```python
from build123d import *

# Parameters (mm, degrees)
F1_DEPTH = 12.7
F2_R     = 2.54
F3_DEPTH = 7.62
F4_R     = 3.175
F5_DEPTH = 2.54


# Not quite as in the source:
# - ends of sketch curves that miss each other by under 0.0002 mm in the source are joined


with BuildPart() as f1:
    # F0 (on Front) → F1 (new body)
    with BuildSketch(Plane.XZ):
        with BuildLine():
            Line((-46.1111856, 159.2312536), (-64.7111856, 159.2312536))
            ThreePointArc((-64.7111856, 159.2312536), (-64.9940283125, 159.1140963125), (-65.1111856, 158.8312536))
            Line((-65.1111856, 158.8312536), (-65.1111856, 157.2332636))
            Line((-65.1111856, 157.2332636), (-64.9611856, 157.2332636))
            Line((-64.9611856, 157.2332636), (-64.9611856, 137.6312536))
            Line((-64.9611856, 137.6312536), (-65.1111856, 137.6312536))
            Line((-65.1111856, 137.6312536), (-65.1111856, 135.7900576))
            ThreePointArc((-65.1111856, 135.7900576), (-65.080737413, 135.6369842271), (-64.9940283125, 135.5072148875))
            Line((-64.9940283125, 135.5072148875), (-63.7917726, 134.3049586))
            Line((-63.7917726, 134.3049586), (-64.1453256, 133.9514056))
            Line((-64.1453256, 133.9514056), (-63.6715641479, 133.4776440521))
            Line((-63.6715641479, 133.4776440521), (-59.6693400521, 129.4754191479))
            Line((-59.6693400521, 129.4754191479), (-59.1955786, 129.0016576))
            Line((-59.1955786, 129.0016576), (-58.8420246, 129.3552116))
            Line((-58.8420246, 129.3552116), (-57.6352246, 128.1484116))
            ThreePointArc((-57.6352246, 128.1484116), (-57.5054559729, 128.061701787), (-57.3523826, 128.0312536))
            Line((-57.3523826, 128.0312536), (-46.1111856, 128.0312536))
            ThreePointArc((-46.1111856, 128.0312536), (-44.6969720376, 128.6170400376), (-44.1111856, 130.0312536))
            Line((-44.1111856, 130.0312536), (-44.1111856, 134.1120546))
            Line((-44.1111856, 134.1120546), (-44.1111856, 153.1264526))
            Line((-44.1111856, 153.1264526), (-44.1111856, 156.3312536))
            Line((-44.1111856, 156.3312536), (-44.1111856, 157.2312536))
            ThreePointArc((-44.1111856, 157.2312536), (-44.6969720376, 158.6454671624), (-46.1111856, 159.2312536))
        make_face()
        with BuildLine():
            Line((-49.0111856, 132.4312536), (-47.1111856, 132.4312536))
            ThreePointArc((-47.1111856, 132.4312536), (-46.0505254282, 131.9919137718), (-45.6111856, 130.9312536))
            ThreePointArc((-45.6111856, 130.9312536), (-46.0505254282, 129.8705934282), (-47.1111856, 129.4312536))
            Line((-47.1111856, 129.4312536), (-49.0111856, 129.4312536))
            ThreePointArc((-49.0111856, 129.4312536), (-50.0718457718, 129.8705934282), (-50.5111856, 130.9312536))
            ThreePointArc((-50.5111856, 130.9312536), (-50.0718457718, 131.9919137718), (-49.0111856, 132.4312536))
        make_face(mode=Mode.SUBTRACT)
        with BuildLine():
            ThreePointArc((-47.1111856, 157.8312536), (-46.0505254282, 157.3919137718), (-45.6111856, 156.3312536))
            ThreePointArc((-45.6111856, 156.3312536), (-46.0505254282, 155.2705934282), (-47.1111856, 154.8312536))
            ThreePointArc((-47.1111856, 154.8312536), (-48.1718457718, 155.2705934282), (-48.6111856, 156.3312536))
            ThreePointArc((-48.6111856, 156.3312536), (-48.1718457718, 157.3919137718), (-47.1111856, 157.8312536))
        make_face(mode=Mode.SUBTRACT)
    extrude(amount=F1_DEPTH)

    # F2 (on face) → F3 (join)
    with BuildSketch(Plane(origin=(34.9030335203, 0, 34.9030264689), x_dir=(0, -1, 0), z_dir=(-0.7071068526, 0, -0.7071067098))):
        with Locations((6.35, 136.8855469037)):
            Circle(F2_R)
    extrude(amount=F3_DEPTH)

    # F4 (on face) → F5 (join)
    with BuildSketch(Plane.YZ.offset(-44.1111856)):
        with Locations((-6.35, 146.5312536)):
            Circle(F4_R)
    extrude(amount=F5_DEPTH)


solid = f1.part
```
Geometry check sheet. Reference: the model listing, model coordinates, mm. A direction names the side the tool comes from. Round coordinates to 2 decimals unless told otherwise and drop trailing zeros. Loops run counter-clockwise (first coordinate to the right, second up) from the corner with the lowest first, then second, coordinate; pieces in that order, holes last. Notation, with made-up numbers: (-15, 23.25) - (29, 23.25) arc R17 ccw to (29, 36.25) - close; hole circle Ø11 at (10.5, 18). An arc over 180 degrees is marked (long way). Write each question's results on one line, items separated by ' | '. Start each with the question number.
Q1. Thickness scan on line 1 (Z direction, x = -46, y = -11.25); line 2 (Z direction, x = -47.75, y = -10.75); line 3 (X direction, y = -11.25, z = 137). Record the ranges inside material, lowest first. Write a range as [from, to].
Q2. Cross-section at C-C on x = -56. Enter the section's corners in (y, z), and give its area (3 significant figures).
Q3. Release check for a two-part mould opening along Z. For faces 1 (the flat face through (-55, -12.7, 144)), 2 (the flat face through (-64.961, -6, 148)), 3 (the flat face through (-55, -6, 159.231)), 4 (the flat face through (-48, -6, 132.431)) record: +Z half, -Z half, draft (parallel to the pull), parting line (faces both ways), or undercut.
Q4. Cross-section at D-D on z = 140. Enter the section's corners in (x, y), and give its area (3 significant figures).
Q5. Cross-section at A-A on x = -47.5. Enter the section's corners in (y, z), and give its area (3 significant figures).
Q6. Cross-section at B-B on z = 145.5. Enter the section's corners in (x, y).
Q7. Access from +Z, -Z, +X, -X, +Y, -Y to the whole of each face (thin tool, end or side, straight path). Record for faces 5 (the cylindrical face through (-42.859, -7.038, 143.432)), 6 (the flat face through (-64.401, -6.261, 134.915)), 7 (the flat face through (-65.111, -6, 158)).
Q8. Gauge pin test, flat ends, axial feed: P1, Ø1, axis at y = -4, z = 132.5, coming from the -X side; P2, Ø6, axis at x = -65, y = -3, coming from the -Z side; P3, Ø4, axis at y = -3.5, z = 150, coming from the -X side. Record the tip position at first contact, or that the pin passes through.
Answers below:
1) line 1: z = [128.03, 129.92], [131.94, 155.32], [157.34, 159.23] | line 2: z = [128.03, 129.43], [132.43, 154.97], [157.69, 159.23] | line 3: x = [-65.11, -44.11]
2) outline: (-12.7, 128.03) - (0, 128.03) - (0, 159.23) - (-12.7, 159.23) - close | area: 396 mm²
3) face 1: draft | face 2: undercut | face 3: +Z half | face 4: undercut
4) outline: (-64.96, -12.7) - (-44.11, -12.7) - (-44.11, 0) - (-64.96, 0) - close | area: 265 mm²
5) outline: (-12.7, 128.03) - (0, 128.03) - (0, 129.43) - (-12.7, 129.43) - close; (-12.7, 132.43) - (0, 132.43) - (0, 154.88) - (-12.7, 154.88) - close; (-12.7, 157.78) - (0, 157.78) - (0, 159.23) - (-12.7, 159.23) - close | area: 321 mm²
6) outline: (-64.96, -12.7) - (-44.11, -12.7) - (-44.11, -9.35) - (-41.57, -9.35) - (-41.57, -3.35) - (-44.11, -3.35) - (-44.11, 0) - (-64.96, 0) - close
7) face 5: +X | face 6: -X, +Y, -Y | face 7: +Z, -X, +Y, -Y
8) P1: stops at x = -63.69 | P2: stops at z = 124.53 | P3: stops at x = -64.96
